Model file for the job. Use its own axes, mm. A direction names the side the tool comes from. Round coordinates to 2 decimals unless told otherwise and drop trailing zeros. Order: outer loops, then holes, each group sorted by start corner. A loop starts at its lowest first (then second) coordinate and runs counter-clockwise, first axis right, second up. Notation, with made-up numbers: (82.5, 6) - (126.5, 6) arc R25 cw to (126.5, 39) - close; hole circle Ø11 at (53.5, -1). An arc over 180 degrees is marked (long way). Put each result on its own line as item: value. Start each with the question number.
Item 1: Saw through at D-D on x = 23. List the corners of the cut face in (y, z) (3 decimals).
Item 2: Pin check, flat tips, straight feed: pin 1 Ø3 at (x, y) = (0, 0) entering from +Z (3 decimals); pin 2 Ø1.5 at (x, y) = (3.5, -21.5) entering from +Z; pin 3 Ø2 at (x, y) = (30, 38) entering from +Z; pin 4 Ø1.5 at (x, z) = (-38.5, -4) entering from +Y. Stop position of each tip, or through.
Item 3: Mould opens along X. For faces 3 (the face through (0, -39, 0)), 4 (the face through (-3, 32, -2.032)), 5 (the face through (-11.012, -49.582, -3.222)), 6 (the face through (-1.58, 0.07, -2.19)) say: pulls with the +X half, pulls with the -X half, needs draft (parallel to the pull), parting line crosses it, or undercut.
Item 4: Saw through at C-C on y = 5. List the corners of the cut face in (x, z) (3 decimals).
Item 5: Saw through at A-A on x = 0. List the corners of the cut face in (y, z) (3 decimals).
Item 6: Saw through at B-B on z = -0.9. List the corners of the cut face in (x, y) (3 decimals).
Item 7: Probe probe 1 along Y at (x, z) = (0, -2.6); probe 2 along X at (y, z) = (-4, -0.45); probe 3 along X at (y, z) = (14.5, -1.25). List the from-to ranges inside material, lowest first.
Item 8: Which spindle directions (+Z, -Z, +X, -X, +Y, -Y) get a long thin tool onto all of the face, cutting with end or side? Do faces 1 (the face through (-1, -11, -4.445)), 2 (the face through (36.946, 11.645, -1.002)). Say none if no direction does.
```python
from build123d import *

# Parameters (mm, degrees)
F0_R     = 50.8
F0_R_2   = 43.815
F0_R_3   = 38.735
F0_R_4   = 31.75
F0_R_5   = 1.581227411
F1_DEPTH = 4.445
F2_DEPTH = 2.032


with BuildPart() as f1:
    # F0 (on Top) → F1 (new body)
    with BuildSketch(Plane.XY):
        with Locations((1.2696e-06, 0.0096165841)):
            Circle(F0_R)
        with Locations((1.2696e-06, 0.0096165841)):
            Circle(F0_R_2, mode=Mode.SUBTRACT)
        with Locations((1.2696e-06, 0.0096165841)):
            Circle(F0_R_2)
        with Locations((1.2696e-06, 0.0096165841)):
            Circle(F0_R_3, mode=Mode.SUBTRACT)
        with Locations((1.2696e-06, 0.0096165841)):
            Circle(F0_R_3)
        with Locations((1.2696e-06, 0.0096165841)):
            Circle(F0_R_4, mode=Mode.SUBTRACT)
        with Locations((1.2696e-06, 0.0096165841)):
            Circle(F0_R_4)
        Circle(F0_R_5, mode=Mode.SUBTRACT)
    extrude(amount=-F1_DEPTH)

    # F0 (on Top) → F2 (cut)
    with BuildSketch(Plane.XY):
        with Locations((1.2696e-06, 0.0096165841)):
            Circle(F0_R)
        with Locations((1.2696e-06, 0.0096165841)):
            Circle(F0_R_2, mode=Mode.SUBTRACT)
        with Locations((1.2696e-06, 0.0096165841)):
            Circle(F0_R_3)
        with Locations((1.2696e-06, 0.0096165841)):
            Circle(F0_R_4, mode=Mode.SUBTRACT)
    extrude(amount=-F2_DEPTH, mode=Mode.SUBTRACT)


solid = f1.part
```
Results found:
1. outline: (-45.285, -4.445) - (45.305, -4.445) - (45.305, -2.032) - (37.302, -2.032) - (37.302, 0) - (31.177, 0) - (31.177, -2.032) - (21.897, -2.032) - (21.897, 0) - (-21.878, 0) - (-21.878, -2.032) - (-31.158, -2.032) - (-31.158, 0) - (-37.283, 0) - (-37.283, -2.032) - (-45.285, -2.032) - close
2. pin 1: passes through
2. pin 2: stops at z = 0
2. pin 3: stops at z = -2.03
2. pin 4: stops at y = 34
3. face 3: needs draft
3. face 4: undercut
3. face 5: parting line crosses it
3. face 6: undercut
4. outline: (-50.554, -4.445) - (50.554, -4.445) - (50.554, -2.032) - (43.53, -2.032) - (43.53, 0) - (38.412, 0) - (38.412, -2.032) - (31.355, -2.032) - (31.355, 0) - (-31.355, 0) - (-31.355, -2.032) - (-38.412, -2.032) - (-38.412, 0) - (-43.53, 0) - (-43.53, -2.032) - (-50.554, -2.032) - close
5. outline: (-50.79, -4.445) - (-1.581, -4.445) - (-1.581, 0) - (-31.74, 0) - (-31.74, -2.032) - (-38.725, -2.032) - (-38.725, 0) - (-43.805, 0) - (-43.805, -2.032) - (-50.79, -2.032) - close; (1.581, -4.445) - (50.81, -4.445) - (50.81, -2.032) - (43.825, -2.032) - (43.825, 0) - (38.745, 0) - (38.745, -2.032) - (31.76, -2.032) - (31.76, 0) - (1.581, 0) - close
6. outline: circle Ø87.63 at (0, 0.01); circle Ø63.5 at (0, 0.01); hole circle Ø77.47 at (0, 0.01); hole circle Ø3.162 at (0, 0)
7. probe 1: y = -50.79 to -1.58, 1.58 to 50.81
7. probe 2: x = -43.63 to -38.53, -31.5 to 31.5, 38.53 to 43.63
7. probe 3: x = -41.35 to -35.92, -28.25 to 28.25, 35.92 to 41.35
8. face 1: -Z, +X, -X, +Y, -Y
8. face 2: +Z
